Check sheet for the modelled part. Datum: model origin and axes. Units: mm. A direction names the side the tool comes from. Give positions to 0.01 mm unless a question says otherwise; leave off trailing zeros. Order: outer loops, then holes, each group sorted by start corner. A loop starts at its lowest first (then second) coordinate and runs counter-clockwise, first axis right, second up. Notation, with made-up numbers: (32.5, 68) - (84.5, 68) arc R15 ccw to (84.5, 85) - close; hole circle Ø3 at (49.25, 79). An arc over 180 degrees is marked (long way). Answer in a Markdown table with one row per item.
Autodesk Inventor part; units mm, degrees
ref_plane "YZ Plane" through (0, 0, 0) normal (1, 0, 0) x (0, 1, 0)
ref_plane "XZ Plane" through (0, 0, 0) normal (0, 1, 0) x (-1, 0, 0)
ref_plane "XY Plane" through (0, 0, 0) normal (0, 0, 1) x (1, 0, 0)
sketch "Sketch1" plane through (0, 0, 0) normal (0, 1, 0) x (-1, 0, 0)
  line L0 (-12.7, 0) -> (12.7, 0)
  line L1 (12.7, 0) -> (12.7, -61.321)
  line L2 (12.7, -61.321) -> (-30.6605, -104.6815)
  line L3 (-30.6605, -104.6815) -> (-48.621, -86.721)
  line L4 (-48.621, -86.721) -> (-12.7, -50.8)
  line L5 (-12.7, -50.8) -> (-12.7, 0)
  point P0 (0, 0)
  point P1 (0, 0)
  dimension "d0" = 25.4
  dimension "d2" = 25.4
  dimension "d4" = 135
  dimension "d8" = 50.8
  dimension "d9" = 50.8
extrude "Extrusion1" add sketch "Sketch1" along normal mid plane 6.35
sketch "Sketch2" plane through (0, 3.175, 0) normal (0, 1, 0) x (1, 0, 0)
  line L0 (12.7, 50.8) -> (12.7, 0) construction
  line L1 (12.7, 0) -> (-12.7, 0) construction
  line L2 (-12.7, 0) -> (-12.7, 61.321) construction
  line L3 (-12.7, 61.321) -> (30.6605, 104.6815) construction
  line L4 (30.6605, 104.6815) -> (48.621, 86.721) construction
  line L5 (48.621, 86.721) -> (12.7, 50.8) construction
  line L6 (48.621, 86.721) -> (30.6605, 104.6815) construction
  line L7 (39.6408, 95.7013) -> (0, 56.0605) construction
  line L8 (0, 56.0605) -> (0, 0) construction
  line L9 (-12.7, 0) -> (12.7, 0) construction
  point P0 (0, 0)
  point P1 (0, 12.7)
  point P2 (0, 38.1)
  point P3 (30.6605, 86.721)
  point P4 (12.7, 68.7605)
  dimension "d12" = 25.4
  dimension "d13" = 12.7
  dimension "d14" = 25.4
  dimension "d15" = 12.7
hole "Hole1" at (0, 3.175, -12.7) at (0, 3.175, -38.1) at (30.6605, 3.175, -86.721) at (12.7, 3.175, -68.7605) direction (0, -1, 0) diameter 5.1054 end through all
fillet "Fillet1" radius 3.302 6 edges at (12.7, 0, -50.8) (-12.7, 0, -61.321) (48.621, 0, -86.721) (30.6605, 0, -104.6815) (12.7, 0, 0) (-12.7, 0, 0)
equation "\"d2\" = d0"
properties part number "CL3-009" material "Aluminum 6061"
(1) Cross-section at D-D, the plane z = -56. Record the cut outline in (x, y) (3 decimals).
Geometry says:
| item | result |
|---|---|
| outline | (-12.7, -3.175) - (17.9, -3.175) - (17.9, 3.175) - (-12.7, 3.175) - close |
(2) Mould release check, pull along X, two halves, no side actions. Record for faces 3 (the cylindrical face through (28.935, -0.044, -88.602)), 4 (the cylindrical face through (-11.707, -0.044, -0.942)), 5 (the cylindrical face through (11.707, 0.044, -0.942)): pulls with the +X half, pulls with the -X half, needs draft (parallel to the pull), parting line crosses it, or undercut.
Geometry says:
| item | result |
|---|---|
| face 3 | undercut |
| face 4 | pulls with the -X half |
| face 5 | pulls with the +X half |
(3) Access from +Z, -Z, +X, -X, +Y, -Y to the whole of each face (thin tool, end or side, straight path). Record for faces 1 (the flat face through (12.7, 0, -27)), 2 (the cylindrical face through (-0.767, -0.044, -10.265)).
Geometry says:
| item | result |
|---|---|
| face 1 | +Z, +X, +Y, -Y |
| face 2 | +Y, -Y |
(4) Cross-section at B-B, the plane y = 2. Record the cut outline in (x, z), then the cut area to 3 significant figures.
Geometry says:
| item | result |
|---|---|
| outline | (-12.7, -59.95) arc R3.3 ccw to (-11.73, -62.29) - (28.33, -102.35) arc R3.3 ccw to (33, -102.35) - (46.29, -89.06) arc R3.3 ccw to (46.29, -84.39) - (13.67, -51.77) arc R3.3 cw to (12.7, -49.43) - (12.7, -3.3) arc R3.3 ccw to (9.4, 0) - (-9.4, 0) arc R3.3 ccw to (-12.7, -3.3) - close; hole circle Ø5.11 at (0, -38.1); hole circle Ø5.11 at (0, -12.7); hole circle Ø5.11 at (12.7, -68.76); hole circle Ø5.11 at (30.66, -86.72) |
| area | 2,760 mm² |
(5) Thickness scan on L1, parallel to X at y = 1, z = -17.5; L2, parallel to Z at x = 1.5, y = 1; L3, parallel to Z at x = 11, y = 2.25. Record the ranges inside material, lowest first.
Geometry says:
| item | result |
|---|---|
| L1 | -12.7 to 12.7 |
| L2 | -75.52 to -40.17, -36.03 to -14.77, -10.63 to 0 |
| L3 | -85.02 to -70.66, -66.86 to -0.41 |
(6) Cross-section at C-C, the plane x = 0. Record the cut outline in (y, z) (3 decimals).
Geometry says:
| item | result |
|---|---|
| outline | (-3.175, -74.021) - (3.175, -74.021) - (3.175, -40.653) - (-3.175, -40.653) - close; (-3.175, -35.547) - (3.175, -35.547) - (3.175, -15.253) - (-3.175, -15.253) - close; (-3.175, -10.147) - (3.175, -10.147) - (3.175, 0) - (-3.175, 0) - close |
(7) Cross-section at A-A, the plane z = -38.1. Record the cut outline in (x, y) (3 decimals), then the cut area to 3 significant figures.
Geometry says:
| item | result |
|---|---|
| outline | (-12.7, -3.175) - (-2.553, -3.175) - (-2.553, 3.175) - (-12.7, 3.175) - close; (2.553, -3.175) - (12.7, -3.175) - (12.7, 3.175) - (2.553, 3.175) - close |
| area | 129 mm² |
(8) Gauge pin test, flat end, axial feed: P1, Ø1.5, axis at y = -1, z = -72, coming from the +X side. Record the tip position at first contact, or that the pin passes through.
Geometry says:
| item | result |
|---|---|
| P1 | x = 34.65 |
